```python
from build123d import *

# Parameters (mm, degrees)
SKETCH_R      = 10
EXTRUDE_DEPTH = 10


with BuildPart() as part:
    # Sketch → Extrude (new body)
    with BuildSketch(Plane.XY):
        with BuildLine():
            ThreePointArc((-10, -38.729833), (0, -40), (10, -38.729833))
            Line((85, -19.364917), (10, -38.729833))
            ThreePointArc((85, -19.364917), (100, 0), (85, 19.364917))
            Line((10, 38.729833), (85, 19.364917))
            ThreePointArc((10, 38.729833), (0, 40), (-10, 38.729833))
            Line((-85, 19.364917), (-10, 38.729833))
            ThreePointArc((-85, 19.364917), (-100, 0), (-85, -19.364917))
            Line((-10, -38.729833), (-85, -19.364917))
        make_face()
        Circle(SKETCH_R, mode=Mode.SUBTRACT)
        with Locations((-80, 0)):
            Circle(SKETCH_R, mode=Mode.SUBTRACT)
        with Locations((80, 0)):
            Circle(SKETCH_R, mode=Mode.SUBTRACT)
    extrude(amount=EXTRUDE_DEPTH)


solid = part.part
```
For this review, take the finished solid that the model builds, in its own axes (mm). Coordinates: 2 decimals unless noted, no trailing zeros. Write each loop counter-clockwise with the first axis right and the second up, starting at its lowest first coordinate (ties: lowest second). Pieces come first, ordered by that corner, then holes. Notation, with made-up numbers: (87, 0.5) -> (130, 0.5) arc R31 ccw to (130, 31.5) -> close; hole circle Ø2 at (25, 57). An arc over 180 degrees is marked (long way). Put each result on its own line as item: value.
Q1. Take a section at B-B, the plane y = 0. State the section outline as (x, z) points, then the cut area to 3 significant figures.
From the geometry:
outline: (-100, 0) -> (-90, 0) -> (-90, 10) -> (-100, 10) -> close; (-70, 0) -> (-10, 0) -> (-10, 10) -> (-70, 10) -> close; (10, 0) -> (70, 0) -> (70, 10) -> (10, 10) -> close; (90, 0) -> (100, 0) -> (100, 10) -> (90, 10) -> close
area: 1,400 mm2
Q2. Take a section at A-A, the plane z = 5. State the section outline as (x, y) points, then the cut area to 3 significant figures.
From the geometry:
outline: (-85, -19.36) -> (-10, -38.73) arc R40 ccw to (10, -38.73) -> (85, -19.36) arc R20 ccw to (85, 19.36) -> (10, 38.73) arc R40 ccw to (-10, 38.73) -> (-85, 19.36) arc R20 ccw to start; hole circle Ø20 at (-80, 0); hole circle Ø20 at (0, 0); hole circle Ø20 at (80, 0)
area: 10,200 mm2
Q3. Clearance check with flat-ended pins moving along their axes: pin 1 Ø23 at (x, y) = (0, 0) entering from -Z; pin 2 Ø1.5 at (x, z) = (-15.5, 6.5) entering from -Y; pin 3 Ø3 at (x, y) = (66, -26.5) entering from +Z. State where each tip first meets the part, or that it passes through.
From the geometry:
pin 1: stops at z = 0
pin 2: stops at y = -37.5
pin 3: passes through
Q4. Take a section at D-D, the plane x = -80. State the section outline as (y, z) points, then the cut area to 3 significant figures.
From the geometry:
outline: (-20.66, 0) -> (-10, 0) -> (-10, 10) -> (-20.66, 10) -> close; (10, 0) -> (20.66, 0) -> (20.66, 10) -> (10, 10) -> close
area: 213 mm2
Q5. The part is to be moulded in two halves that separate along X. For faces 1 (the cylindrical face through (-2.17, -9.76, 4.93)), 2 (the flat face through (-48.025, 28.912, 4.93)), 3 (the cylindrical face through (70, 0, 5)), 4 (the cylindrical face through (0, -40, 5)), say which applies: +X half, -X half, draft (parallel to the pull), parting line (faces both ways), or undercut.
From the geometry:
face 1: undercut
face 2: -X half
face 3: undercut
face 4: parting line
Q6. Wall thickness on L1, parallel to X at y = -5, z = 2.25; L2, parallel to X at y = -3, z = 8.25; L3, parallel to Y at x = 80, z = 5: over which ranges is each line inside the solid? List them lowest first.
From the geometry:
L1: x = -99.36 to -88.66, -71.34 to -8.66, 8.66 to 71.34, 88.66 to 99.36
L2: x = -99.77 to -89.54, -70.46 to -9.54, 9.54 to 70.46, 89.54 to 99.77
L3: y = -20.66 to -10, 10 to 20.66
Q7. Take a section at C-C, the plane x = 0. State the section outline as (y, z) points.
From the geometry:
outline: (-40, 0) -> (-10, 0) -> (-10, 10) -> (-40, 10) -> close; (10, 0) -> (40, 0) -> (40, 10) -> (10, 10) -> close
